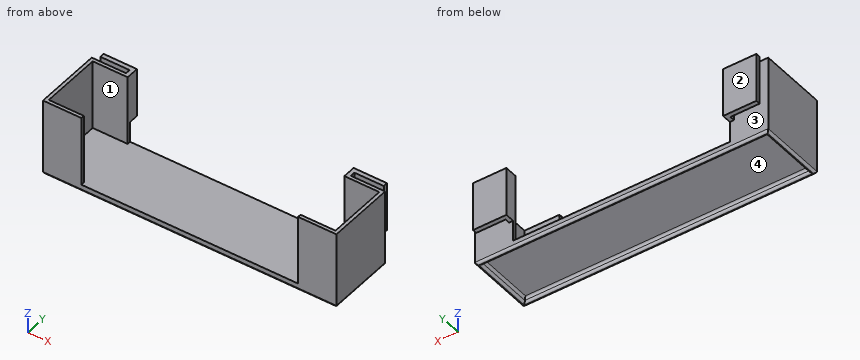
from build123d import *

# Parameters (mm, degrees)
ESQUISSE1_W        = 130
ESQUISSE1_H        = 30
BOSS_EXTRU_1_DEPTH = 1
BOSS_EXTRU_2_DEPTH = 31
ESQUISSE5_W        = 1.8
ESQUISSE5_H        = 21.8
BOSS_EXTRU_4_DEPTH = 2.2
ESQUISSE6_W        = 14.8
ESQUISSE6_H        = 21.8
BOSS_EXTRU_5_DEPTH = 2
ESQUISSE3_W        = 130
ESQUISSE3_H        = 30
ESQUISSE3_W_2      = 126
ESQUISSE3_H_2      = 26
BOSS_EXTRU_3_DEPTH = 2
CONG_1_R           = 1


with BuildPart() as part:
    # Esquisse1 → Boss.-Extru.1 (new body)
    with BuildSketch(Plane.XY):
        with Locations((65, 15)):
            Rectangle(ESQUISSE1_W, ESQUISSE1_H)
    extrude(amount=BOSS_EXTRU_1_DEPTH)

    # Esquisse2 → Boss.-Extru.2 (add)
    with BuildSketch(Plane.XY.offset(1)):
        Polygon((128.5, 28.5), (113, 28.5), (113, 30), (130, 30), (130, 0), (113, 0), (113, 1.5), (128.5, 1.5), align=None)
        Polygon((1.5, 28.5), (1.5, 1.5), (17, 1.5), (17, 0), (0, 0), (0, 30), (17, 30), (17, 28.5), align=None)
    extrude(amount=BOSS_EXTRU_2_DEPTH)

    # Esquisse5 → Boss.-Extru.4 (add)
    with BuildSketch(Plane(origin=(0, 30, 0), x_dir=(1, 0, 0), z_dir=(0, 1, 0))):
        with Locations((16.1, -21.1)):
            Rectangle(ESQUISSE5_W, ESQUISSE5_H)
        with Locations((113.9, -21.1)):
            Rectangle(ESQUISSE5_W, ESQUISSE5_H)
    extrude(amount=BOSS_EXTRU_4_DEPTH)

    # Esquisse6 → Boss.-Extru.5 (add)
    with BuildSketch(Plane(origin=(0, 32.2, 0), x_dir=(1, 0, 0), z_dir=(0, 1, 0))):
        with Locations((9.6, -21.1)):
            Rectangle(ESQUISSE6_W, ESQUISSE6_H)
        with Locations((120.4, -21.1)):
            Rectangle(ESQUISSE6_W, ESQUISSE6_H)
    extrude(amount=BOSS_EXTRU_5_DEPTH)

    # Esquisse3 → Boss.-Extru.3 (add)
    with BuildSketch(Plane(origin=(0, 0, 0), x_dir=(-1, 0, 0), z_dir=(0, 0, -1))):
        with Locations((-65, 15)):
            Rectangle(ESQUISSE3_W, ESQUISSE3_H)
        with Locations((-65, 15)):
            Rectangle(ESQUISSE3_W_2, ESQUISSE3_H_2, mode=Mode.SUBTRACT)
    extrude(amount=BOSS_EXTRU_3_DEPTH)

    # Congé1
    cong_1_edges = [part.edges().sort_by_distance(p)[0] for p in [
        (65, 28, 0),
        (2, 15, 0),
        (65, 2, 0),
        (128, 15, 0),
        (2, 15, -2),
        (65, 28, -2),
        (128, 15, -2),
        (65, 2, -2),
        (130, 15, -2),
        (65, 30, -2),
        (0, 15, -2),
        (65, 0, -2),
    ]]
    fillet(cong_1_edges, radius=CONG_1_R - 0.0001)  # a hair under: the kernel refuses the full size


solid = part.part
Verification items for the finished model (mm, model axes). Face numbers are marked on the shaded views. A direction names the side the tool comes from. Round coordinates to 2 decimals unless told otherwise and drop trailing zeros. Loops run counter-clockwise (first coordinate to the right, second up) from the corner with the lowest first, then second, coordinate; pieces in that order, holes last. Notation, with made-up numbers: (-3, 40.25) - (14, 40.25) arc R14 cw to (14, 62.25) - close; hole circle Ø3 at (42.5, -34). An arc over 180 degrees is marked (long way). Use one line per item in the form item = value.
1. Section check A-A on z = 2.5. Record the cut outline in (x, y).
A:
outline = (0, 0) - (17, 0) - (17, 1.5) - (1.5, 1.5) - (1.5, 28.5) - (17, 28.5) - (17, 30) - (0, 30) - close; (113, 0) - (130, 0) - (130, 30) - (113, 30) - (113, 28.5) - (128.5, 28.5) - (128.5, 1.5) - (113, 1.5) - close
2. Scan lines: probe 1 along Y at (x, z) = (14.5, 28.5); probe 2 along X at (y, z) = (22, 16); probe 3 along X at (y, z) = (33, 25). Record each from-to range of solid material in increasing order.
A:
probe_1 = 0 to 1.5, 28.5 to 30, 32.2 to 34.2
probe_2 = 0 to 1.5, 128.5 to 130
probe_3 = 2.2 to 17, 113 to 127.8
3. Access from +Z, -Z, +X, -X, +Y, -Y to the whole of each face (thin tool, end or side, straight path). Record for the marked faces 1 and 2.
A:
face_1 = +Z
face_2 = +Z, -Z, +X, -X, +Y
4. Draft check along Z on the marked faces 3 and 4. Enter one of: pulls with the +Z half, pulls with the -Z half, needs draft (parallel to the pull), parting line crosses it, or undercut.
A:
face_3 = needs draft
face_4 = pulls with the -Z half
5. Gauge pin test, flat ends, axial feed: pin 1 Ø0.6 at (y, z) = (33, 17) entering from -X; pin 2 Ø1.1 at (y, z) = (31.5, 16.5) entering from +X; pin 3 Ø4 at (x, z) = (69, 4) entering from -Y; pin 4 Ø8 at (x, y) = (49, 18) entering from -Z. Record the tip position at first contact, or that the pin passes through.
A:
pin_1 = 2.2
pin_2 = 114.8
pin_3 = through
pin_4 = 0
